Verification items for the finished model (mm, model axes). Face numbers are marked on the shaded views. Coordinates: 2 decimals unless noted, no trailing zeros. Write each loop counter-clockwise with the first axis right and the second up, starting at its lowest first coordinate (ties: lowest second). Pieces come first, ordered by that corner, then holes. Notation, with made-up numbers: (21.25, 45.5) -> (32.25, 45.5) arc R22 cw to (32.25, 56.5) -> close; hole circle Ø6 at (83.5, 42). An arc over 180 degrees is marked (long way). Answer in a Markdown table with one row per item.
```python
from build123d import *

# Parameters (mm, degrees)
BOSS_EXTRU_1_DEPTH      = 70
ESQUISSE3_W             = 1
ESQUISSE3_H             = 4
BOSS_EXTRU_2_DEPTH      = 3
ESQUISSE4_W             = 1
ESQUISSE4_H             = 4
BOSS_EXTRU_3_DEPTH      = 3
ESQUISSE6_R             = 0.75
ENL_V_MAT_EXTRU_1_DEPTH = 5
ESQUISSE7_W             = 4
ESQUISSE7_H             = 1
BOSS_EXTRU_4_DEPTH      = 3
ESQUISSE8_W             = 4
ESQUISSE8_H             = 1
BOSS_EXTRU_5_DEPTH      = 3
ESQUISSE9_R             = 0.75
ENL_V_MAT_EXTRU_2_DEPTH = 5.1
ESQUISSE10_W            = 4
ESQUISSE10_H            = 1
BOSS_EXTRU_6_DEPTH      = 3
ESQUISSE11_W            = 4
ESQUISSE11_H            = 1
BOSS_EXTRU_7_DEPTH      = 3
ESQUISSE12_R            = 0.75
ENL_V_MAT_EXTRU_3_DEPTH = 5.1
ESQUISSE13_W            = 11
ESQUISSE13_H            = 11
BOSS_EXTRU_8_DEPTH      = 3


with BuildPart() as part:
    # Esquisse1 → Boss.-Extru.1 (new body)
    with BuildSketch(Plane.XY):
        Polygon((-1.402144657, 1.200833509), (1.095290548, -3.130773283), (3.597855343, 1.200833509), align=None)
    extrude(amount=BOSS_EXTRU_1_DEPTH)

    # Esquisse3 → Boss.-Extru.2 (add)
    with BuildSketch(Plane(origin=(0, 1.200833509, 0), x_dir=(1, 0, 0), z_dir=(0, 1, 0))):
        with Locations((-0.902144657, -30)):
            Rectangle(ESQUISSE3_W, ESQUISSE3_H)
    extrude(amount=BOSS_EXTRU_2_DEPTH)

    # Esquisse4 → Boss.-Extru.3 (add)
    with BuildSketch(Plane(origin=(0, 1.200833509, 0), x_dir=(1, 0, 0), z_dir=(0, 1, 0))):
        with Locations((3.097855343, -30)):
            Rectangle(ESQUISSE4_W, ESQUISSE4_H)
    extrude(amount=BOSS_EXTRU_3_DEPTH)

    # Esquisse6 → Enlèv. mat.-Extru.1 (cut)
    with BuildSketch(Plane(origin=(3.597855343, 0, 0), x_dir=(0, 0, -1), z_dir=(1, 0, 0))):
        with Locations(Location((-30, 2.950833509, 0), (0, 0, 90))):
            Circle(ESQUISSE6_R)
    extrude(amount=-ENL_V_MAT_EXTRU_1_DEPTH, mode=Mode.SUBTRACT)

    # Esquisse7 → Boss.-Extru.4 (add)
    with BuildSketch(Plane(origin=(2.177314873, -1.257933098, 0), x_dir=(0, 0, -1), z_dir=(0.8658773126093765, -0.5002564137603478, 0))):
        with Locations((-29.999890103, 2.339624703)):
            Rectangle(ESQUISSE7_W, ESQUISSE7_H)
    extrude(amount=BOSS_EXTRU_4_DEPTH)

    # Esquisse8 → Boss.-Extru.5 (add)
    with BuildSketch(Plane(origin=(2.177314873, -1.257933098, 0), x_dir=(0, 0, -1), z_dir=(0.8658773126093764, -0.5002564137603477, 0))):
        with Locations((-29.999890103, -1.662939435)):
            Rectangle(ESQUISSE8_W, ESQUISSE8_H)
    extrude(amount=BOSS_EXTRU_5_DEPTH)

    # Esquisse9 → Enlèv. mat.-Extru.2 (cut)
    with BuildSketch(Plane(origin=(-1.082024325, -1.872840185, 0), x_dir=(-0.8658773126093765, 0.5002564137603478, 0), z_dir=(-0.5002564137603477, -0.8658773126093764, 0))):
        with Locations(Location((-4.264576651, -29.999890103, 0), (0, 0, 180))):
            Circle(ESQUISSE9_R)
    extrude(amount=-ENL_V_MAT_EXTRU_2_DEPTH, mode=Mode.SUBTRACT)

    # Esquisse10 → Boss.-Extru.6 (add)
    with BuildSketch(Plane(origin=(-0.532707143, -0.307138122, 0), x_dir=(0, 0, 1), z_dir=(-0.8663213583248282, -0.499487040983272, 0))):
        with Locations((29.999890103, -2.759339198)):
            Rectangle(ESQUISSE10_W, ESQUISSE10_H)
    extrude(amount=BOSS_EXTRU_6_DEPTH)

    # Esquisse11 → Boss.-Extru.7 (add)
    with BuildSketch(Plane(origin=(-0.532707143, -0.307138122, 0), x_dir=(0, 0, 1), z_dir=(-0.8663213583248282, -0.499487040983272, 0))):
        with Locations((30, 1.240660802)):
            Rectangle(ESQUISSE11_W, ESQUISSE11_H)
    extrude(amount=BOSS_EXTRU_7_DEPTH)

    # Esquisse12 → Enlèv. mat.-Extru.3 (cut)
    with BuildSketch(Plane(origin=(-0.869437513, 1.50797163, 0), x_dir=(0.866321358324828, 0.499487040983272, 0), z_dir=(-0.499487040983272, 0.866321358324828, 0))):
        with Locations(Location((-2.364907088, -30, 0), (0, 0, 180))):
            Circle(ESQUISSE12_R)
    extrude(amount=-ENL_V_MAT_EXTRU_3_DEPTH, mode=Mode.SUBTRACT)

    # Esquisse13 → Boss.-Extru.8 (add)
    with BuildSketch(Plane.XY.offset(70)):
        with Locations((1.097855343, -0.880773283)):
            Rectangle(ESQUISSE13_W, ESQUISSE13_H)
    extrude(amount=BOSS_EXTRU_8_DEPTH)


solid = part.part
```
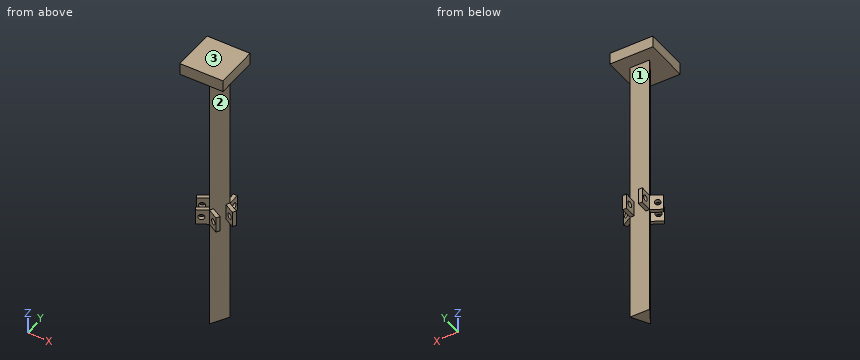
1. Sectioned sample at A-A, the plane z = 8. Record the cut outline in (x, y), and give its area (3 significant figures).
Findings below:
| item | result |
|---|---|
| outline | (-1.4, 1.2) -> (1.1, -3.13) -> (3.6, 1.2) -> close |
| area | 10.8 mm² |
2. Go/stop test with flat-tipped pins: pin 1 (5.5 mm diameter, centred on x = 2, z = 20.5, fed in from +Y); pin 2 (6 mm diameter, centred on y = 3, z = 51.5, fed in from +X); pin 3 (0.5 mm diameter, centred on x = 3, z = 30.5, fed in from +Y). Record where each tip stops, or that it passes through.
Findings below:
| item | result |
|---|---|
| pin 1 | stops at y = 1.2 |
| pin 2 | stops at x = 3.6 |
| pin 3 | stops at y = 4.2 |
3. Material ranges on probe 1 along Z at (x, y) = (3.25, 3.75); probe 2 along Z at (x, y) = (2.25, -3.5); probe 3 along X at (y, z) = (1.5, 30.5), recorded low to high. Write a range as from..to.
Findings below:
| item | result |
|---|---|
| probe 1 | z = 28..32, 70..73 |
| probe 2 | z = 28..29.51, 30.49..32, 70..73 |
| probe 3 | x = -1.4..-0.4, 2.6..3.6 |
4. Release check for a two-part mould opening along Z. For the marked faces 1, 2 and 3 record: released by +Z, released by -Z, zero draft, split by the parting line, or undercut.
Findings below:
| item | result |
|---|---|
| face 1 | undercut |
| face 2 | undercut |
| face 3 | released by +Z |
